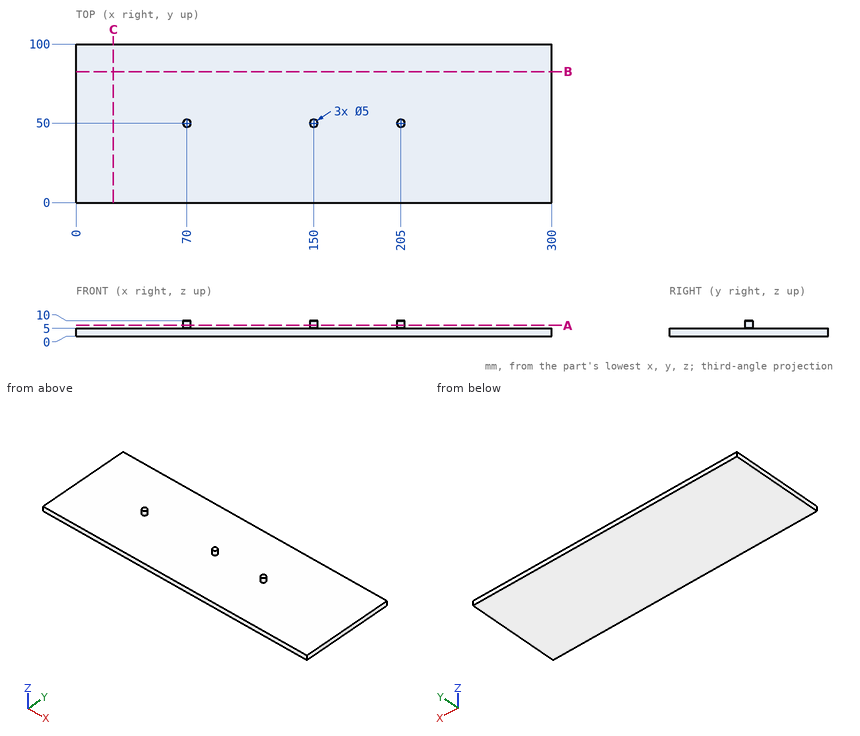
For this review, use the dimensioned drawing (mm, ordinates from the lowest corner) and the shaded views. Give positions to 0.01 mm unless a question says otherwise; leave off trailing zeros. Write each loop counter-clockwise with the first axis right and the second up, starting at its lowest first coordinate (ties: lowest second). Pieces come first, ordered by that corner, then holes. Notation, with made-up numbers: M 53.5,-33 L 59.5,-33 A27 ccw 59.5,-3 Z; hole C 59,67 d9. An arc over 180 degrees is marked long. Answer as a JSON object with one key per item and string values. Group by question number.
Item 1: Consider section A-A on z = 7. Write out the cut boundary in (x, y).
Item 2: For pin 1 Ø1 at (x, y) = (69, 21.5) entering from +Z, flat-tipped, find the tip position at first contact; note if it passes through.
Item 3: For probe 1 along X at (y, z) = (52, 8); probe 2 along Z at (x, y) = (209.5, 50.5); probe 3 along Y at (x, z) = (148, 9.25), list the stretches that pass through material, from the lowest coordinate up. Write a range as [from, to].
Item 4: Consider section C-C on x = 23.5. Write out the cut boundary in (y, z).
Item 5: Consider section B-B on y = 82.5. Write out the cut boundary in (x, z).
Check result:
{
 "1": {"outline": "C 70,50 d5; C 150,50 d5; C 205,50 d5"},
 "2": {"pin 1": "stops at z = 5"},
 "3": {"probe 1": "x = [68.5, 71.5], [148.5, 151.5], [203.5, 206.5]", "probe 2": "z = [0, 5]", "probe 3": "y = [48.5, 51.5]"},
 "4": {"outline": "M 0,0 L 100,0 L 100,5 L 0,5 Z"},
 "5": {"outline": "M 0,0 L 300,0 L 300,5 L 0,5 Z"}
}
